Solid Edge part; units mm, degrees
sketch "Sketch1" plane through (0, 0, 0) normal (0, -1, 0) x (1, 0, 0)
  line L0 (22.5, 0) -> (32.5, 42)
  line L1 (26.3323, 42) -> (32.5, 42)
  line L2 (19.1894, 12) -> (26.3323, 42)
  line L3 (11.25, 12) -> (19.1894, 12)
  line L4 (11.25, 0) -> (11.25, 12)
  line L5 (11.25, 0) -> (22.5, 0)
revolve "RevolvedProtrusion1" add sketch "Sketch1" angle 360 about axis through (0, 0, 0) along (0, 0, 1)
sketch "Sketch2" plane through (0, 0, 0) normal (0, -1, 0) x (1, 0, 0)
  circle A0 centre (0, 42) radius 5
extrude "Cutout1" cut sketch "Sketch2" along normal through all and the other way through all
sketch "Sketch3" plane through (0, 0, 0) normal (1, 0, 0) x (0, 1, 0)
  circle A0 centre (-0.0054, 42.0317) radius 5
extrude "Cutout2" cut sketch "Sketch3" along normal through all and the other way through all
Source: CAD feature listing. Evaluate the final solid. Frame: model axes, mm. A direction names the side the tool comes from. Give positions to 0.01 mm unless a question says otherwise; leave off trailing zeros. Loops run counter-clockwise (first coordinate to the right, second up) from the corner with the lowest first, then second, coordinate; pieces in that order, holes last. Notation, with made-up numbers: (50, -19) -> (86, -19) arc R10 cw to (86, -15) -> close; hole circle Ø6 at (17, -5.75). An arc over 180 degrees is marked (long way). Use a Markdown table: item, result. Add a question column.
1) Section query D-D, the plane z = 35.5. Return the cut outline in (x, y).
2) Section query C-C, the plane z = 27. Return the cut outline in (x, y), then the cut area to 3 significant figures.
3) Pull-direction query (X, two-part tool) for faces 3 (the face through (0, 29, 37)), 4 (the face through (24.441, -10.134, 16.627)), 5 (the face through (19, 20, 42)); classes: +X half, -X half, draft (parallel to the pull), parting line (faces both ways), or undercut.
4) Section query B-B, the plane y = 0. Return the cut outline in (x, z).
5) Reachability of faces 1 (the face through (28.583, 0.104, 37.033)), 2 (the face through (8.3, -8.3, 12)) from +Z, -Z, +X, -X, +Y, -Y: full face, straight path, thin tool, end or side. Return the list, or none.
6) Section query A-A, the plane x = 0. Return the cut outline in (y, z).
7) First-contact query: pin 1 (19 mm diameter, centred on x = -2.5, y = -7, fed in from +Z); pin 2 (5 mm diameter, centred on x = -18, z = 10, fed in from -Y); pin 3 (18 mm diameter, centred on x = 0, y = 0, fed in from -Z); pin 4 (3 mm diameter, centred on x = 22.5, z = 9, fed in from +Y). Flat tips, straight axial feed; report the tip coordinate or a pass-through.
8) Line query: line 1 along Y through (x, z) = (0, 6); line 2 along Z through (x, y) = (-7, -12.5); line 3 along Y through (x, z) = (-19.5, 29). Output: solid intervals per line, ascending. Write a range as [from, to].
Numbers:
| question | item | result |
|---|---|---|
| 1 | outline | circle Ø61.9 at (0, 0); hole circle Ø49.57 at (0, 0) |
| 2 | outline | circle Ø57.86 at (0, 0); hole circle Ø45.52 at (0, 0) |
| 2 | area | 1,000 mm2 |
| 3 | face 3 | undercut |
| 3 | face 4 | parting line |
| 3 | face 5 | draft |
| 4 | outline | (-31.32, 37.03) -> (-22.5, 0) -> (-11.25, 0) -> (-11.25, 12) -> (-19.19, 12) -> (-25.15, 37.03) -> close; (11.25, 0) -> (22.5, 0) -> (31.32, 37.03) -> (25.15, 37.03) -> (19.19, 12) -> (11.25, 12) -> close |
| 5 | face 1 | +Z, +X, -X |
| 5 | face 2 | +Z |
| 6 | outline | (-31.31, 37) -> (-22.5, 0) -> (-11.25, 0) -> (-11.25, 12) -> (-19.19, 12) -> (-25.14, 37) -> close; (11.25, 0) -> (22.5, 0) -> (31.31, 37) -> (25.14, 37) -> (19.19, 12) -> (11.25, 12) -> close |
| 7 | pin 1 | stops at z = 12 |
| 7 | pin 2 | stops at y = -19.6 |
| 7 | pin 3 | passes through |
| 7 | pin 4 | stops at y = 12.99 |
| 8 | line 1 | y = [-23.93, -11.25], [11.25, 23.93] |
| 8 | line 2 | z = [0, 12] |
| 8 | line 3 | y = [-22.01, -12.64], [12.64, 22.01] |
